Check sheet for the modelled part. Datum: model origin and axes. Units: mm. A direction names the side the tool comes from. Round coordinates to 2 decimals unless told otherwise and drop trailing zeros. Order: outer loops, then holes, each group sorted by start corner. A loop starts at its lowest first (then second) coordinate and runs counter-clockwise, first axis right, second up. Notation, with made-up numbers: (-7.75, 68) -> (42.25, 68) arc R26 ccw to (42.25, 101) -> close; hole circle Ø1 at (-38.75, 63). An arc over 180 degrees is marked (long way). Answer in a Markdown table with one row per item.
from build123d import *

# Parameters (mm, degrees)
BOSS_EXTRU_1_DEPTH      = 20
D_GAGEMENT_M2_51_D      = 2.9
ENL_V_MAT_EXTRU_1_DEPTH = 14
D_GAGEMENT_M31_D        = 3.4
CONG_1_R                = 2


with BuildPart() as part:
    # Esquisse1 → Boss.-Extru.1 (new body)
    with BuildSketch(Plane.XY):
        with BuildLine():
            Line((-5.5, 0), (-5.5, 8.076655966))
            Line((-5.5, 8.076655966), (-2.5, 8.076655966))
            Line((-2.5, 8.076655966), (-2.5, 2.076655966))
            ThreePointArc((-2.5, 2.076655966), (0, -3.25), (2.5, 2.076655966))
            Line((2.5, 2.076655966), (2.5, 8.076655966))
            Line((2.5, 8.076655966), (5.5, 8.076655966))
            Line((5.5, 8.076655966), (5.5, 0))
            ThreePointArc((5.5, 0), (4.91934955, -2.459674775), (3.3, -4.4))
            ThreePointArc((3.3, -4.4), (2.711145618, -5.105572809), (2.5, -6))
            Line((2.5, -6), (2.5, -8))
            ThreePointArc((2.5, -8), (1.914213562, -9.414213562), (0.5, -10))
            Line((0.5, -10), (-0.5, -10))
            ThreePointArc((-0.5, -10), (-1.914213562, -9.414213562), (-2.5, -8))
            Line((-2.5, -8), (-2.5, -6))
            ThreePointArc((-2.5, -6), (-2.711145618, -5.105572809), (-3.3, -4.4))
            ThreePointArc((-3.3, -4.4), (-4.91934955, -2.459674775), (-5.5, 0))
        make_face()
    extrude(amount=BOSS_EXTRU_1_DEPTH)

    # Dégagement M2.51 (through all)
    with Locations(Plane(origin=(5.5, 0, 0), x_dir=(0, 0, -1), z_dir=(1, 0, 0))):
        with Locations((-10, 5.576655966)):
            Hole(D_GAGEMENT_M2_51_D / 2)

    # Esquisse5 → Enlèv. mat.-Extru.1 (cut)
    with BuildSketch(Plane(origin=(0, 0, 0), x_dir=(-1, 0, 0), z_dir=(0, 0, -1))):
        with BuildLine():
            Line((-2.5, -6), (-2.5, -8))
            ThreePointArc((-2.5, -8), (-1.914213562, -9.414213562), (-0.5, -10))
            Line((-0.5, -10), (0.5, -10))
            ThreePointArc((0.5, -10), (1.914213562, -9.414213562), (2.5, -8))
            Line((2.5, -8), (2.5, -6))
            ThreePointArc((2.5, -6), (2.711145618, -5.105572809), (3.3, -4.4))
            Line((3.3, -4.4), (-3.3, -4.4))
            ThreePointArc((-3.3, -4.4), (-2.711145618, -5.105572809), (-2.5, -6))
        make_face()
    extrude(amount=-ENL_V_MAT_EXTRU_1_DEPTH, mode=Mode.SUBTRACT)

    # Dégagement M31 (through all)
    with Locations(Plane(origin=(0, -7.5, 20), x_dir=(1, 0, 0), z_dir=(0, 0, 1))):
        with Locations((0, 0)):
            Hole(D_GAGEMENT_M31_D / 2)

    # Congé1
    cong_1_edges = [part.edges().sort_by_distance(p)[0] for p in [
        (-2.5, 2.076655966, 10),
        (2.5, 2.076655966, 10),
    ]]
    fillet(cong_1_edges, radius=CONG_1_R)


solid = part.part
Item 1: Cross-section at C-C (y = -7.5). Record the boundary of the cut face in (x, z).
Result sheet:
| item | result |
|---|---|
| outline | (-2.5, 14) -> (-1.7, 14) -> (-1.7, 20) -> (-2.5, 20) -> close; (1.7, 14) -> (2.5, 14) -> (2.5, 20) -> (1.7, 20) -> close |
Item 2: Mould release check, pull along Y, two halves, no side actions. Record for faces 1 (the flat face through (2.5, 3.6, 9.9)), 2 (the cylindrical face through (-1.9, -9.43, 16.96)), 3 (the cylindrical face through (0.37, -9.16, 16.96)): pulls with the +Y half, pulls with the -Y half, needs draft (parallel to the pull), parting line crosses it, or undercut.
Result sheet:
| item | result |
|---|---|
| face 1 | needs draft |
| face 2 | pulls with the -Y half |
| face 3 | undercut |
Item 3: Cross-section at D-D (z = 18.5). Record the boundary of the cut face in (x, y), and give its area (3 significant figures).
Result sheet:
| item | result |
|---|---|
| outline | (-5.5, 0) arc R5.5 ccw to (-3.3, -4.4) arc R2 cw to (-2.5, -6) -> (-2.5, -8) arc R2 ccw to (-0.5, -10) -> (0.5, -10) arc R2 ccw to (2.5, -8) -> (2.5, -6) arc R2 cw to (3.3, -4.4) arc R5.5 ccw to (5.5, 0) -> (5.5, 8.08) -> (2.5, 8.08) -> (2.5, 2.7) arc R2 ccw to (2.79, 1.67) arc R3.25 cw (long way) to (-2.79, 1.67) arc R2 ccw to (-2.5, 2.7) -> (-2.5, 8.08) -> (-5.5, 8.08) -> close; hole circle Ø3.4 at (0, -7.5) |
| area | 90.2 mm^2 |
Item 4: Scan lines: line 1 (Y direction, x = 0, z = 16.55); line 2 (X direction, y = 5, z = 14); line 3 (X direction, y = 1.25, z = 17). Record each from-to range of solid material in increasing order. Write a range as [from, to].
Result sheet:
| item | result |
|---|---|
| line 1 | y = [-10, -9.2], [-5.8, -3.25] |
| line 2 | x = [-5.5, -2.5], [2.5, 5.5] |
| line 3 | x = [-5.5, -3], [3, 5.5] |
Item 5: Cross-section at A-A (z = 10). Record the boundary of the cut face in (x, y), and give its area (3 significant figures).
Result sheet:
| item | result |
|---|---|
| outline | (-5.5, 0) arc R5.5 ccw to (-3.3, -4.4) -> (3.3, -4.4) arc R5.5 ccw to (5.5, 0) -> (5.5, 4.13) -> (2.5, 4.13) -> (2.5, 2.7) arc R2 ccw to (2.79, 1.67) arc R3.25 cw (long way) to (-2.79, 1.67) arc R2 ccw to (-2.5, 2.7) -> (-2.5, 4.13) -> (-5.5, 4.13) -> close; (-5.5, 7.03) -> (-2.5, 7.03) -> (-2.5, 8.08) -> (-5.5, 8.08) -> close; (2.5, 7.03) -> (5.5, 7.03) -> (5.5, 8.08) -> (2.5, 8.08) -> close |
| area | 54.8 mm^2 |
Item 6: Set-up check for faces 4 (the flat face through (0, -5, 14)), 5 (the flat face through (-2.5, 3.6, 9.9)), 6 (the cylindrical face through (2.57, 2.18, 10.14)): record each of +Z, -Z, +X, -X, +Y, -Y from which the full face is reachable in a straight line by a thin tool's end or side.
Result sheet:
| item | result |
|---|---|
| face 4 | -Z, +X, -X, -Y |
| face 5 | +Z, -Z, +Y |
| face 6 | +Z, -Z |
Item 7: Depth check by flat-ended pin: P1, Ø3, axis at x = -1.5, y = -6, coming from the -Z side; P2, Ø3, axis at y = -6.5, z = 16, coming from the +X side; P3, Ø1.6, axis at y = -7, z = 17.5, coming from the -X side. Enter the tip coordinate at first touch or a pass-through.
Result sheet:
| item | result |
|---|---|
| P1 | stops at z = 14 |
| P2 | stops at x = 2.77 |
| P3 | stops at x = -2.5 |
Item 8: Cross-section at B-B (x = 0). Record the boundary of the cut face in (y, z), and give its area (3 significant figures).
Result sheet:
| item | result |
|---|---|
| outline | (-10, 14) -> (-9.2, 14) -> (-9.2, 20) -> (-10, 20) -> close; (-5.8, 14) -> (-4.4, 14) -> (-4.4, 0) -> (-3.25, 0) -> (-3.25, 20) -> (-5.8, 20) -> close |
| area | 36.2 mm^2 |
